```python
from build123d import *

# Parameters (mm, degrees)
F0_W     = 13
F0_H     = 4
F0_W_2   = 12
F1_DEPTH = 4
F2_DEPTH = 9
F4_DEPTH = 4


with BuildPart() as f1:
    # F0 (on Top) → F1 (new body)
    with BuildSketch(Plane.XY):
        with Locations((6.5, 2)):
            Rectangle(F0_W, F0_H)
        with Locations((19, 2)):
            Rectangle(F0_W_2, F0_H)
        with Locations((31.5, 2)):
            Rectangle(F0_W, F0_H)
        with Locations((44, 2)):
            Rectangle(F0_W_2, F0_H)
        with Locations((56.5, 2)):
            Rectangle(F0_W, F0_H)
        with Locations((69, 2)):
            Rectangle(F0_W_2, F0_H)
        with Locations((81.5, 2)):
            Rectangle(F0_W, F0_H)
        with Locations((94, 2)):
            Rectangle(F0_W_2, F0_H)
        with Locations((106.5, 2)):
            Rectangle(F0_W, F0_H)
        with Locations((119, 2)):
            Rectangle(F0_W_2, F0_H)
        with Locations((131.5, 2)):
            Rectangle(F0_W, F0_H)
        with Locations((144, 2)):
            Rectangle(F0_W_2, F0_H)
        with Locations((156.5, 2)):
            Rectangle(F0_W, F0_H)
    extrude(amount=F1_DEPTH)

    # F0 (on Top) → F2 (join)
    with BuildSketch(Plane.XY):
        with Locations((6.5, 2)):
            Rectangle(F0_W, F0_H)
        with Locations((31.5, 2)):
            Rectangle(F0_W, F0_H)
        with Locations((56.5, 2)):
            Rectangle(F0_W, F0_H)
        with Locations((81.5, 2)):
            Rectangle(F0_W, F0_H)
        with Locations((106.5, 2)):
            Rectangle(F0_W, F0_H)
        with Locations((131.5, 2)):
            Rectangle(F0_W, F0_H)
        with Locations((156.5, 2)):
            Rectangle(F0_W, F0_H)
    extrude(amount=F2_DEPTH)

    # F3 (on face) → F4 (join)
    with BuildSketch(Plane.XZ):
        Polygon((13, 0), (0, 0), (6.5, -13.518506), align=None)
        Polygon((38, 0), (25, 0), (31.5, -13.518506), align=None)
        Polygon((63, 0), (50, 0), (56.5, -13.518506), align=None)
        Polygon((88, 0), (75, 0), (81.5, -13.518506), align=None)
        Polygon((113, 0), (100, 0), (106.5, -13.518506), align=None)
        Polygon((138, 0), (125, 0), (131.5, -13.518506), align=None)
        Polygon((163, 0), (150, 0), (156.5, -13.518506), align=None)
    extrude(amount=-F4_DEPTH)


solid = f1.part
```
For this review, take the finished solid that the model builds, in its own axes (mm). A direction names the side the tool comes from. Give positions to 0.01 mm unless a question says otherwise; leave off trailing zeros. Write each loop counter-clockwise with the first axis right and the second up, starting at its lowest first coordinate (ties: lowest second). Pieces come first, ordered by that corner, then holes.
Item 1: Take a section at D-D (x = 29). Give the boundary of the cut face in (y, z).
Item 2: Take a section at C-C (z = -4.25). Give the boundary of the cut face in (x, y).
Item 3: Take a section at A-A (z = -11.25). Give the boundary of the cut face in (x, y), and give its area (3 significant figures).
Item 4: Take a section at B-B (x = 93). Give the boundary of the cut face in (y, z), and give its area (3 significant figures).
Item 5: Wall thickness on probe 1 along Z at (x, y) = (65, 1.35); probe 2 along Z at (x, y) = (34, 2.95): over which ranges is each line inside the solid? List them lowest first.
Item 6: Insertion check: P1, Ø1.2, axis at x = 119, y = 3, coming from the -Z side; P2, Ø1.2, axis at x = 117, y = 1.5, coming from the +Z side; P3, Ø1.5, axis at y = 2, z = -3.5, coming from the +X side. Each pin has a flat end and moves straight along its axis. Give the tip position at first contact, or say it passes through.
Item 7: Machinability: for faces 3 (the face through (75, 2, 6)), 4 (the face through (103.204, 1.972, -6.665)), 5 (the face through (156, 2, 9)), which of the approach directions +Z, -Z, +X, -X, +Y, -Y give a long, thin tool a straight path to every point of the face, cutting with its end or side? Answer none if there is none.
Item 8: The part is to be moulded in two halves that separate along X. For faces 1 (the face through (6, 2, 9)), 2 (the face through (144, 2, 4)), say which applies: +X half, -X half, draft (parallel to the pull), parting line (faces both ways), or undercut.
Established:
1. outline: (0, -8.32) - (4, -8.32) - (4, 9) - (0, 9) - close
2. outline: (2.04, 0) - (10.96, 0) - (10.96, 4) - (2.04, 4) - close; (27.04, 0) - (35.96, 0) - (35.96, 4) - (27.04, 4) - close; (52.04, 0) - (60.96, 0) - (60.96, 4) - (52.04, 4) - close; (77.04, 0) - (85.96, 0) - (85.96, 4) - (77.04, 4) - close; (102.04, 0) - (110.96, 0) - (110.96, 4) - (102.04, 4) - close; (127.04, 0) - (135.96, 0) - (135.96, 4) - (127.04, 4) - close; (152.04, 0) - (160.96, 0) - (160.96, 4) - (152.04, 4) - close
3. outline: (5.41, 0) - (7.59, 0) - (7.59, 4) - (5.41, 4) - close; (30.41, 0) - (32.59, 0) - (32.59, 4) - (30.41, 4) - close; (55.41, 0) - (57.59, 0) - (57.59, 4) - (55.41, 4) - close; (80.41, 0) - (82.59, 0) - (82.59, 4) - (80.41, 4) - close; (105.41, 0) - (107.59, 0) - (107.59, 4) - (105.41, 4) - close; (130.41, 0) - (132.59, 0) - (132.59, 4) - (130.41, 4) - close; (155.41, 0) - (157.59, 0) - (157.59, 4) - (155.41, 4) - close
3. area: 61.1 mm2
4. outline: (0, 0) - (4, 0) - (4, 4) - (0, 4) - close
4. area: 16.0 mm2
5. probe 1: z = 0 to 4
5. probe 2: z = -8.32 to 9
6. P1: stops at z = 0
6. P2: stops at z = 4
6. P3: stops at x = 161.68
7. face 3: +Z, +Y, -Y
7. face 4: -Z, +Y, -Y
7. face 5: +Z, +X, -X, +Y, -Y
8. face 1: draft
8. face 2: undercut
